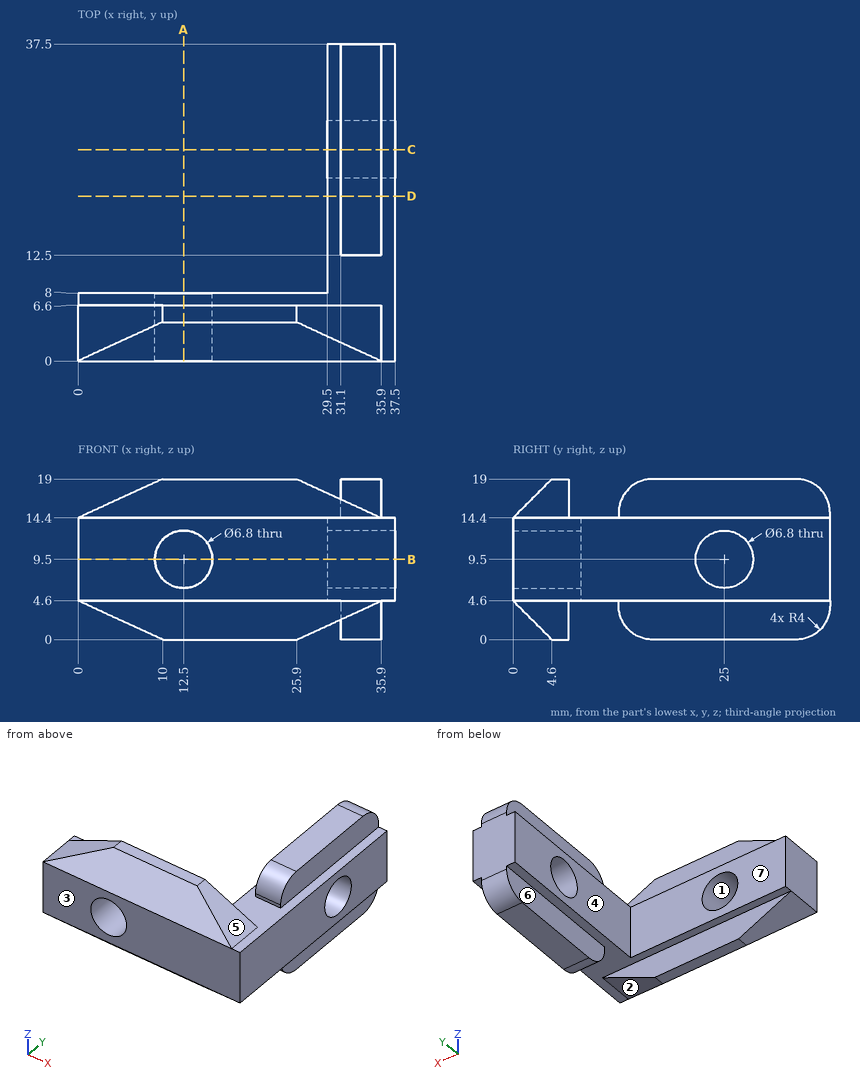
Print and shaded views of the part. All mm, measured from the part's lowest x, y and z. A direction names the side the tool comes from. Coordinates: 2 decimals unless noted, no trailing zeros. Loops run counter-clockwise (first coordinate to the right, second up) from the corner with the lowest first, then second, coordinate; pieces in that order, holes last. Notation, with made-up numbers: (-37, 37.5) - (19, 37.5) arc R11 cw to (19, 47.5) - close; hole circle Ø11 at (64.25, -5.5). An arc over 180 degrees is marked (long way). Write item = value, one per line. Start each with the question number.
Item 1: Cut at A-A, the plane x = 12.5. Give the cut face in (y, z).
Item 2: 3-axis set-ups, long thin cutter, end or side, ignore diameter. For the marked faces 5, 6 and 7: which of +Z, -Z, +X, -X, +Y, -Y reach the whole face in a straight line?
Item 3: Cut at B-B, the plane z = 9.5. Give the cut face in (x, y), and give its area (3 significant figures).
Item 4: Cut at C-C, the plane y = 25. Give the cut face in (x, z).
Item 5: Cut at D-D, the plane y = 19.5. Give the cut face in (x, z), and give its area (3 significant figures).
Item 6: Wall check: L1, parallel to Y at x = 35.5, z = 9.5; L2, parallel to X at y = 2, z = 9.5; L3, parallel to Y at x = 13, z = 13.75. Give the ranges that are in metal, low to high. Write a range as from..to.
Item 7: Mould opens along X. For the marked faces 1, 2, 3 and 4 say: released by +X, released by -X, zero draft, split by the parting line, or undercut.
Item 8: Flat gauge pins, fed straight in: pin 1 Ø1.4 at (y, z) = (29, 2.5) entering from +X; pin 2 Ø1.4 at (y, z) = (24, 3) entering from -X; pin 3 Ø8 at (x, z) = (12.5, 9.5) entering from +Y; pin 4 Ø2 at (y, z) = (10.5, 3) entering from +X. Where does each tip first touch, or does it go through?
The answers:
q1.outline = (0, 4.6) - (4.6, 0) - (6.6, 0) - (6.6, 4.6) - (8, 4.6) - (8, 6.1) - (0, 6.1) - close; (0, 12.9) - (8, 12.9) - (8, 14.4) - (6.6, 14.4) - (6.6, 19) - (4.6, 19) - (0, 14.4) - close
q2.face_5 = +Z, +X, -Y
q2.face_6 = -Z, -X, +Y
q2.face_7 = +Z, -Z, -X, +Y
q3.outline = (0, 0) - (9.1, 0) - (9.1, 8) - (0, 8) - close; (15.9, 0) - (37.5, 0) - (37.5, 21.6) - (29.5, 21.6) - (29.5, 8) - (15.9, 8) - close; (29.5, 28.4) - (37.5, 28.4) - (37.5, 37.5) - (29.5, 37.5) - close
q3.area = 427 mm2
q4.outline = (29.5, 4.6) - (31.1, 4.6) - (31.1, 0) - (35.9, 0) - (35.9, 4.6) - (37.5, 4.6) - (37.5, 6.1) - (29.5, 6.1) - close; (29.5, 12.9) - (37.5, 12.9) - (37.5, 14.4) - (35.9, 14.4) - (35.9, 19) - (31.1, 19) - (31.1, 14.4) - (29.5, 14.4) - close
q5.outline = (29.5, 4.6) - (31.1, 4.6) - (31.1, 0) - (35.9, 0) - (35.9, 4.6) - (37.5, 4.6) - (37.5, 14.4) - (35.9, 14.4) - (35.9, 19) - (31.1, 19) - (31.1, 14.4) - (29.5, 14.4) - close
q5.area = 123 mm2
q6.L1 = 0..21.6, 28.4..37.5
q6.L2 = 0..9.1, 15.9..37.5
q6.L3 = 0..8
q7.face_1 = undercut
q7.face_2 = released by +X
q7.face_3 = zero draft
q7.face_4 = released by -X
q8.pin_1 = 35.9
q8.pin_2 = 31.1
q8.pin_3 = 8
q8.pin_4 = through
